Can you work these out from the model? Positions are in its coordinate system, mm. A direction names the side the tool comes from. Give positions to 0.01 mm unless a question says otherwise; leave off trailing zeros. Order: outer loops, then holes, each group sorted by start corner. A loop starts at its lowest first (then second) coordinate and runs counter-clockwise, first axis right, second up. Notation, with made-up numbers: M 88.5,88 L 114.5,88 A15 cw 114.5,105 Z; hole C 80,25.25 d5. An arc over 180 degrees is marked long. Answer as a JSON object with one key per item and string values.
```python
from build123d import *

# Parameters (mm, degrees)
SKETCH1_W           = 25.4
SKETCH1_H           = 25.4
BOSS_EXTRUDE1_DEPTH = 12.7
HOLE1_D             = 6.5278
HOLE1_DEPTH         = 100
HOLE1_CBORE_D       = 10.3124
HOLE1_CBORE_DEPTH   = 22.225
HOLE2_D             = 6.5278
HOLE2_DEPTH         = 100
HOLE2_CBORE_D       = 10.3124
HOLE2_CBORE_DEPTH   = 22.225
HOLE3_D             = 6.5278
HOLE3_DEPTH         = 100
HOLE3_CBORE_D       = 10.3124
HOLE3_CBORE_DEPTH   = 22.225
SKETCH8_W           = 6.1976
SKETCH8_H           = 2.9718
BOSS_EXTRUDE2_DEPTH = 2.2098
CIRPATTERN1_COUNT   = 2
CIRPATTERN1_ANGLE   = 270
SKETCH9_W           = 6.1976
SKETCH9_H           = 2.9718
BOSS_EXTRUDE3_DEPTH = 2.2098
CIRPATTERN2_COUNT   = 2
CIRPATTERN2_ANGLE   = 270
SKETCH10_W          = 2.9718
SKETCH10_H          = 6.1976
BOSS_EXTRUDE4_DEPTH = 2.2098
CIRPATTERN3_COUNT   = 2
CIRPATTERN3_ANGLE   = 90
CHAMFER1_SIZE       = 0.635


with BuildPart() as part:
    # Sketch1 → Boss-Extrude1 (new, symmetric)
    with BuildSketch(Plane.XY):
        Rectangle(SKETCH1_W, SKETCH1_H)
    extrude(amount=BOSS_EXTRUDE1_DEPTH, both=True)

    # Hole1
    with Locations(Plane.XY.offset(12.7)):
        with Locations((0, 0)):
            CounterBoreHole(HOLE1_D / 2, HOLE1_CBORE_D / 2, HOLE1_CBORE_DEPTH, depth=HOLE1_DEPTH)

    # Hole2
    with Locations(Plane(origin=(12.7, 0, 0), x_dir=(0, 0, -1), z_dir=(1, 0, 0))):
        with Locations((0, 0)):
            CounterBoreHole(HOLE2_D / 2, HOLE2_CBORE_D / 2, HOLE2_CBORE_DEPTH, depth=HOLE2_DEPTH)

    # Hole3
    with Locations(Plane.XZ.offset(12.7)):
        with Locations((0, 0)):
            CounterBoreHole(HOLE3_D / 2, HOLE3_CBORE_D / 2, HOLE3_CBORE_DEPTH, depth=HOLE3_DEPTH)

    # Sketch8 → Boss-Extrude2 (add)
    with BuildSketch(Plane(origin=(0, 12.7, 0), x_dir=(1, 0, 0), z_dir=(0, 1, 0))):
        with Locations((0, 11.2141)):
            Rectangle(SKETCH8_W, SKETCH8_H)
    boss_extrude2 = extrude(amount=BOSS_EXTRUDE2_DEPTH)

    # CirPattern1: Boss-Extrude2 ×2 about axis
    cirpattern1_axis = Axis((0, 0, 0), (0, -1, 0))
    for i in range(1, CIRPATTERN1_COUNT):
        add(boss_extrude2.rotate(cirpattern1_axis, i * CIRPATTERN1_ANGLE / (CIRPATTERN1_COUNT - 1)))

    # Sketch9 → Boss-Extrude3 (add)
    with BuildSketch(Plane.ZY.offset(12.7)):
        with Locations((0, 11.2141)):
            Rectangle(SKETCH9_W, SKETCH9_H)
    boss_extrude3 = extrude(amount=BOSS_EXTRUDE3_DEPTH)

    # CirPattern2: Boss-Extrude3 ×2 about axis
    cirpattern2_axis = Axis((0, 0, 0), (1, 0, 0))
    for i in range(1, CIRPATTERN2_COUNT):
        add(boss_extrude3.rotate(cirpattern2_axis, i * CIRPATTERN2_ANGLE / (CIRPATTERN2_COUNT - 1)))

    # Sketch10 → Boss-Extrude4 (add)
    with BuildSketch(Plane(origin=(0, 0, -12.7), x_dir=(-1, 0, 0), z_dir=(0, 0, -1))):
        with Locations((11.2141, 0)):
            Rectangle(SKETCH10_W, SKETCH10_H)
    boss_extrude4 = extrude(amount=BOSS_EXTRUDE4_DEPTH)

    # CirPattern3: Boss-Extrude4 ×2 about axis
    cirpattern3_axis = Axis((0, 0, 0), (0, 0, -1))
    for i in range(1, CIRPATTERN3_COUNT):
        add(boss_extrude4.rotate(cirpattern3_axis, i * CIRPATTERN3_ANGLE / (CIRPATTERN3_COUNT - 1)))

    # Chamfer1
    chamfer1_edges = [part.edges().sort_by_distance(p)[0] for p in [
        (0, -12.7, 12.7),
        (12.7, 0, 12.7),
        (12.7, -12.7, 0),
    ]]
    chamfer(chamfer1_edges, length=CHAMFER1_SIZE)


solid = part.part
```
1) For faces 1 (the face through (-14, 11, 3.099)), 2 (the face through (-7.198, 3.485, 3.8)), 3 (the face through (-14, 11, -3.099)), 4 (the face through (-9.728, 14, 0)), 5 (the face through (-3.8, 7.198, 3.485)), which set-ups out of +Z, -Z, +X, -X, +Y, -Y let a thin tool reach every point of the face, with its end or its side?
Results found:
{"face 1": "+Z, -X, +Y, -Y", "face 2": "+X", "face 3": "-Z, -X, +Y, -Y", "face 4": "+Z, -Z, +X, +Y", "face 5": "-Y"}
2) I want a section at A-A on z = 0. Count the separate pieces of the cut face and the enclosed holes in it, and give its area (3 significant figures).
Results found:
{"separate pieces": "4", "enclosed holes": "0", "area": "265 mm²"}
3) I need wall thicknesses on L1, parallel to Y at x = -6.45, z = 0; L2, parallel to Z at x = -0.25, y = 9.25; L3, parallel to Y at x = -10.6, z = 0. Which ranges of each line are inside material? Lowest first, please.
Results found:
{"L1": "y = -12.7 to -5.16, 5.16 to 12.7", "L2": "z = -12.7 to -5.15, 5.15 to 12.7", "L3": "y = -12.7 to -3.26, 3.26 to 14.91"}
4) I want a section at B-B on x = -10.75. Write out the boundary of the cut face in (y, z) (3 decimals), and give its area (3 significant figures).
Results found:
{"outline": "M -12.7,-12.7 L -3.099,-12.7 L -3.099,-14.91 L 3.099,-14.91 L 3.099,-12.7 L 12.7,-12.7 L 12.7,-3.099 L 14.91,-3.099 L 14.91,3.099 L 12.7,3.099 L 12.7,12.7 L -12.065,12.7 L -12.7,12.065 Z; hole C 0,0 d6.528", "area": "639 mm²"}
5) I'm going to push flat-ended pins straight in: pin 1 Ø1.8 at (x, z) = (-11, -14) entering from +Y; pin 2 Ø3 at (y, z) = (-5, 8) entering from -X; pin 3 Ø2.5 at (x, y) = (-13.5, 10.5) entering from -Z; pin 4 Ø8 at (y, z) = (1, -8) entering from -X. Where does each tip first touch, or does it pass through?
Results found:
{"pin 1": "stops at y = 3.1", "pin 2": "stops at x = -12.7", "pin 3": "stops at z = -12.7", "pin 4": "stops at x = -14.91"}
6) I want a section at C-C on y = 12.25. Write out the boundary of the cut face in (x, z) (3 decimals), and give its area (3 significant figures).
Results found:
{"outline": "M -14.91,-3.099 L -12.7,-3.099 L -12.7,-12.7 L -3.099,-12.7 L -3.099,-14.91 L 3.099,-14.91 L 3.099,-12.7 L 12.7,-12.7 L 12.7,12.065 L 12.065,12.7 L -12.7,12.7 L -12.7,3.099 L -14.91,3.099 Z; hole C 0,0 d6.528", "area": "639 mm²"}
7) Thinking about a two-plate mould opening in Y: for faces 6 (the face through (-9.728, 0, -14)), 7 (the face through (0.708, -3.186, -11.135)), 8 (the face through (8.24, 0.23, 5.15)), 9 (the face through (-14, 9.728, 0)), which applies, pulls with the +Y half, pulls with the -Y half, needs draft (parallel to the pull), parting line crosses it, or undercut?
Results found:
{"face 6": "needs draft", "face 7": "undercut", "face 8": "undercut", "face 9": "pulls with the -Y half"}
